Model file for the job. Use its own axes, mm. Round coordinates to 2 decimals unless told otherwise and drop trailing zeros. Loops run counter-clockwise (first coordinate to the right, second up) from the corner with the lowest first, then second, coordinate; pieces in that order, holes last. Notation, with made-up numbers: M -27,19.5 L 2,19.5 A19 cw 2,43.5 Z; hole C 65.5,31.5 d8. An arc over 180 degrees is marked long. Use a Markdown table: item, result. Add a question column.
Item 1: Pin check, flat tips, straight feed: P1, Ø1.5, axis at y = 1, z = 18.5, coming from the +X side; P2, Ø1, axis at x = 1, z = 2.5, coming from the -Y side; P3, Ø2, axis at x = 1, z = 6, coming from the -Y side. Stop position of each tip, or through.
Item 2: Wall check: L1, parallel to Z at x = 0.5, y = -1.4; L2, parallel to Y at x = -0.05, z = 1; L3, parallel to Z at x = 1.4, y = -0.8. Give the ranges that are in metal, low to high. Write a range as from..to.
Item 3: Saw through at C-C on z = 7. Write the cut outline in (x, y), then the cut area to 3 significant figures.
Item 4: Saw through at A-A on x = 0. Write the cut outline in (y, z).
Autodesk Inventor part; units mm, degrees
ref_plane "YZ Plane" through (0, 0, 0) normal (1, 0, 0) x (0, 1, 0)
ref_plane "XZ Plane" through (0, 0, 0) normal (0, 1, 0) x (-1, 0, 0)
ref_plane "XY Plane" through (0, 0, 0) normal (0, 0, 1) x (1, 0, 0)
sketch "Sketch1" plane through (0, 0, 0) normal (0, 0, 1) x (1, 0, 0)
  circle A0 centre (0, 0) radius 1
  circle A1 centre (0, 0) radius 1.75
  dimension "d0" = 2
  dimension "d1" = 3.5
extrude "Extrusion1" add sketch "Sketch1" along normal blind 30 contours A0
extrude "Extrusion2" add sketch "Sketch1" against normal blind 1.5 contours A0 | A1
sketch "Sketch2" plane through (0, 0, 30) normal (0, 0, 1) x (1, 0, 0)
  circle A0 centre (0, 0) radius 1.75
  circle A1 centre (0, 0) radius 1
  circle A2 centre (0, 0) radius 1
extrude "Extrusion3" add sketch "Sketch2" along normal blind 1.5 contours A0 | A1
chamfer "Chamfer1" distance 0.25 angle 45 4 edges at (-1.75, 0, 31.5) (-1.75, 0, -1.5) (-1.75, 0, 30) (-1.75, 0, 0)
properties part number "CNCT_STEEL_Outlet_door_hinge_pin" material "Stainless Steel"
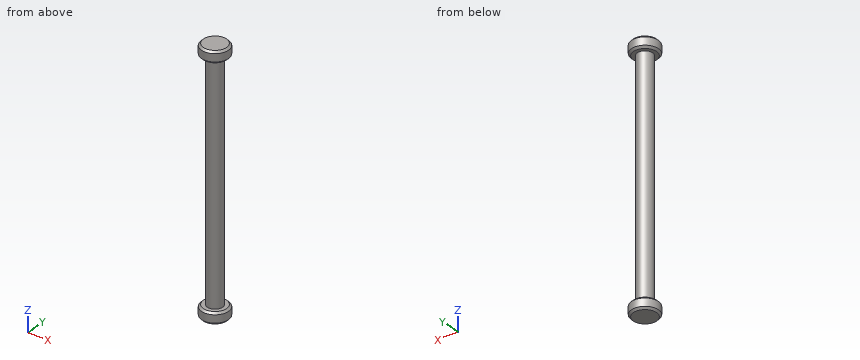
Entries:
| question | item | result |
|---|---|---|
| 1 | P1 | x = 0.97 |
| 1 | P2 | y = -0.87 |
| 1 | P3 | y = -1 |
| 2 | L1 | -1.5..0, 30..31.5 |
| 2 | L2 | -1..1 |
| 2 | L3 | -1.39..-0.11, 30.11..31.39 |
| 3 | outline | C 0,0 d2 |
| 3 | area | 3.14 mm2 |
| 4 | outline | M -1.75,-1.25 L -1.5,-1.5 L 1.5,-1.5 L 1.75,-1.25 L 1.75,-0.25 L 1.5,0 L 1,0 L 1,30 L 1.5,30 L 1.75,30.25 L 1.75,31.25 L 1.5,31.5 L -1.5,31.5 L -1.75,31.25 L -1.75,30.25 L -1.5,30 L -1,30 L -1,0 L -1.5,0 L -1.75,-0.25 Z |
